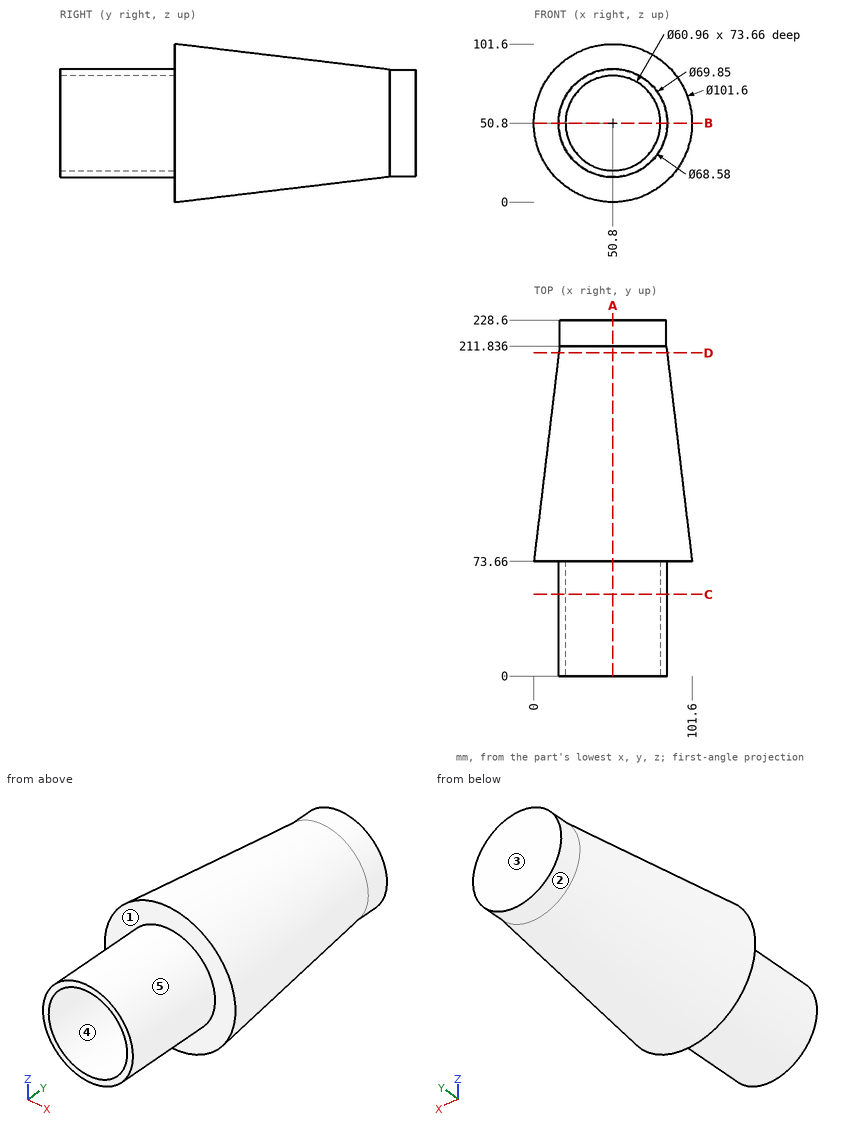
Verification items for this drawing (mm, ordinates from the low corner). A direction names the side the tool comes from. Give positions to 0.01 mm unless a question says otherwise; leave off trailing zeros. Write each loop counter-clockwise with the first axis right and the second up, starting at its lowest first coordinate (ties: lowest second). Pieces come first, ordered by that corner, then holes. Notation, with made-up numbers: (29, 46.5) - (87, 46.5) arc R21 ccw to (87, 68.5) - close; hole circle Ø10 at (-7.5, -36). An arc over 180 degrees is marked (long way). Answer as CSV lines item,"result". Start each with the question number.
1. Sectioned sample at C-C (y = 52.5). Record the boundary of the cut face in (x, z) (3 decimals).
2. Sectioned sample at B-B (z = 50.8). Record the boundary of the cut face in (x, y) (3 decimals), then the cut area to 3 significant figures.
3. Set-up check for the marked faces 1 and 2: record each of +Z, -Z, +X, -X, +Y, -Y from which the full face is reachable in a straight line by a thin tool's end or side.
4. Thickness scan on line 1 (X direction, y = 20.5, z = 50.8) (3 decimals); line 2 (Z direction, x = 50, y = 18); line 3 (Y direction, x = 80, z = 57.5). Record the ranges inside material, lowest first.
5. Draft check along X on the marked faces 3, 4 and 5. Enter one of: pulls with the +X half, pulls with the -X half, needs draft (parallel to the pull), parting line crosses it, or undercut.
6. Sectioned sample at A-A (x = 50.8). Record the boundary of the cut face in (y, z) (3 decimals).
7. Depth check by flat-ended pin: pin 1 (1.5 mm diameter, centred on x = 70.5, y = 154.5, fed in from +Z); pin 2 (3 mm diameter, centred on y = 189.5, z = 63, fed in from +X); pin 3 (8 mm diameter, centred on x = 82, z = 76, fed in from -Y). Enter the tip coordinate at first touch or a pass-through.
8. Sectioned sample at D-D (y = 207.5). Record the boundary of the cut face in (x, z).
Derived:
1,outline,"circle Ø69.85 at (50.8, 50.8); hole circle Ø60.96 at (50.8, 50.8)"
2,outline,"(0, 73.66) - (15.875, 73.66) - (15.875, 0) - (20.32, 0) - (20.32, 73.66) - (81.28, 73.66) - (81.28, 0) - (85.725, 0) - (85.725, 73.66) - (101.6, 73.66) - (85.09, 211.836) - (85.09, 228.6) - (16.51, 228.6) - (16.51, 211.836) - close"
2,area,"13,600 mm²"
3,face 1,"-Y"
3,face 2,"+Y"
4,line 1,"15.875 to 20.32, 81.28 to 85.725"
4,line 2,"15.88 to 20.33, 81.27 to 85.72"
4,line 3,"73.66 to 228.6"
5,face 3,"needs draft"
5,face 4,"undercut"
5,face 5,"parting line crosses it"
6,outline,"(0, 15.875) - (73.66, 15.875) - (73.66, 0) - (211.836, 16.51) - (228.6, 16.51) - (228.6, 85.09) - (211.836, 85.09) - (73.66, 101.6) - (73.66, 85.725) - (0, 85.725) - (0, 81.28) - (73.66, 81.28) - (73.66, 20.32) - (0, 20.32) - close"
7,pin 1,"z = 87.33"
7,pin 2,"x = 86.21"
7,pin 3,"y = 73.66"
8,outline,"circle Ø69.62 at (50.8, 50.8)"
